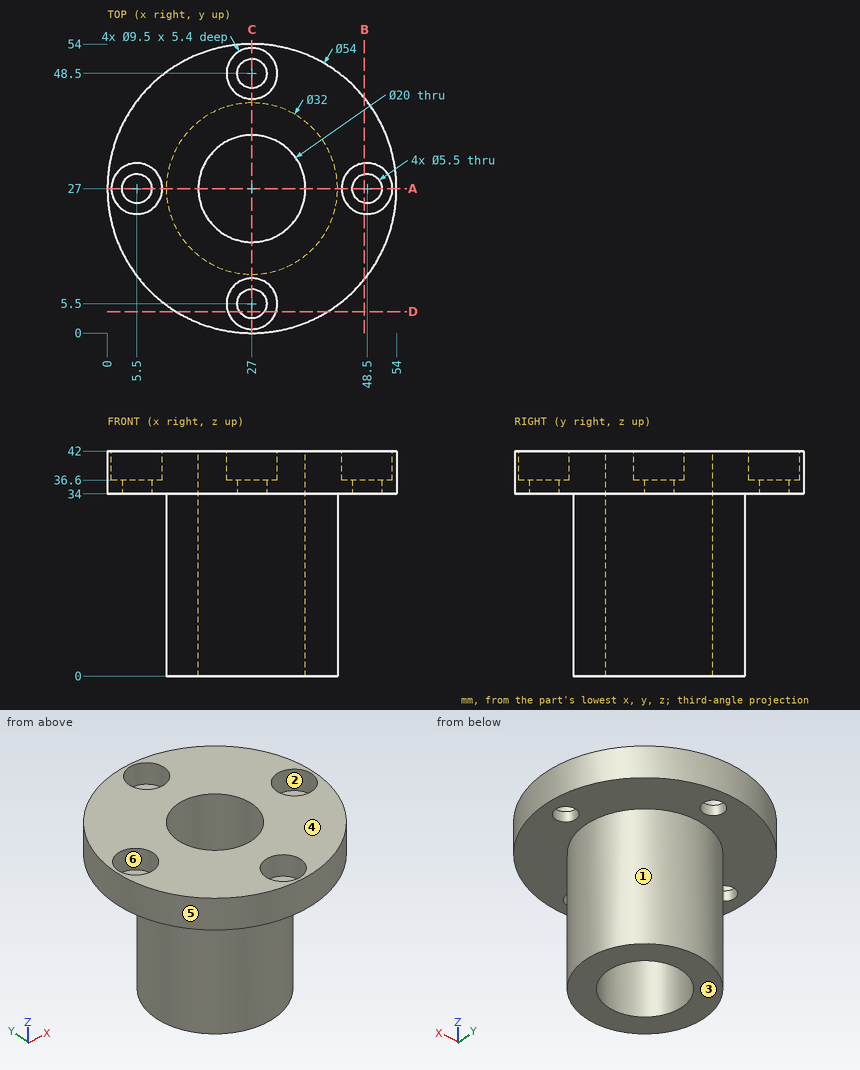
Design review of the part shown in the three views and the two pictorial views. Dimensions are in mm from the part's minimum x, y and z. A direction names the side the tool comes from. Round coordinates to 2 decimals unless told otherwise and drop trailing zeros. Order: outer loops, then holes, each group sorted by start corner. A loop starts at its lowest first (then second) coordinate and runs counter-clockwise, first axis right, second up.
Q1. Insertion check: P1, Ø1, axis at x = 39.5, z = 16, coming from the +Y side; P2, Ø4, axis at x = 41.5, z = 19, coming from the -Y side; P3, Ø3, axis at x = 25.5, z = 37.5, coming from the -Y side. Each pin has a flat end and moves straight along its axis. Give the tip position at first contact, or say it passes through.
Findings below:
P1: stops at y = 37.58
P2: stops at y = 17.01
P3: stops at y = 0
Q2. Mouldability with a two-part tool opening along Y and no side actions: class the marked faces 4, 5 and 6 as pulls with the +Y half, pulls with the -Y half, needs draft (parallel to the pull), parting line crosses it, or undercut.
Findings below:
face 4: needs draft
face 5: parting line crosses it
face 6: undercut
Q3. We need section B-B, the plane x = 48. Give the boundary of the cut face in (y, z), plus the area to 3 significant figures.
Findings below:
outline: (10.03, 34) - (24.3, 34) - (24.3, 36.6) - (22.28, 36.6) - (22.28, 42) - (10.03, 42) - close; (29.7, 34) - (43.97, 34) - (43.97, 42) - (31.72, 42) - (31.72, 36.6) - (29.7, 36.6) - close
area: 206 mm2
Q4. Machinability: for the marked faces 1, 2 and 3, which of the approach directions +Z, -Z, +X, -X, +Y, -Y give a long, thin tool a straight path to every point of the face, cutting with its end or side? Answer none if there is none.
Findings below:
face 1: -Z
face 2: +Z
face 3: -Z, +X, -X, +Y, -Y
Q5. Wall thickness on line 1 (Y direction, x = 27, z = 35.1); line 2 (X direction, y = 5, z = 40); line 3 (X direction, y = 31, z = 36.5): over which ranges is each line inside the solid? List them lowest first.
Findings below:
line 1: y = 0 to 2.75, 8.25 to 17, 37 to 45.75, 51.25 to 54
line 2: x = 11.35 to 22.28, 31.72 to 42.65
line 3: x = 0.3 to 17.83, 36.17 to 53.7
Q6. We need section A-A, the plane y = 27. Give the boundary of the cut face in (x, z), plus the area to 3 significant figures.
Findings below:
outline: (0, 34) - (2.75, 34) - (2.75, 36.6) - (0.75, 36.6) - (0.75, 42) - (0, 42) - close; (8.25, 34) - (11, 34) - (11, 0) - (17, 0) - (17, 42) - (10.25, 42) - (10.25, 36.6) - (8.25, 36.6) - close; (37, 0) - (43, 0) - (43, 34) - (45.75, 34) - (45.75, 36.6) - (43.75, 36.6) - (43.75, 42) - (37, 42) - close; (51.25, 34) - (54, 34) - (54, 42) - (53.25, 42) - (53.25, 36.6) - (51.25, 36.6) - close
area: 549 mm2
Q7. We need section D-D, the plane y = 4. Give the boundary of the cut face in (x, z).
Findings below:
outline: (12.86, 34) - (24.7, 34) - (24.7, 36.6) - (22.49, 36.6) - (22.49, 42) - (12.86, 42) - close; (29.3, 34) - (41.14, 34) - (41.14, 42) - (31.51, 42) - (31.51, 36.6) - (29.3, 36.6) - close
